Read the model definition and answer for the solid it produces. Units are mm, in the model's axes. A direction names the side the tool comes from. Give positions to 0.01 mm unless a question says otherwise; leave off trailing zeros. Write each loop counter-clockwise with the first axis right and the second up, starting at its lowest first coordinate (ties: lowest second). Pieces come first, ordered by that corner, then holes.
Solid Edge part; units mm, degrees
sketch "Sketch1" plane through (0, 0, 0) normal (0, 0, 1) x (1, 0, 0)
  circle A0 centre (0, 0) radius 41.05
  circle A1 centre (0, 0) radius 20.625
  circle A2 centre (159.79, 0) radius 23.37
  circle A3 centre (159.79, 0) radius 10
extrude "Protrusion1" add sketch "Sketch1" along normal blind 17.73
sketch "Sketch2" plane through (0, 0, 0) normal (0, 0, 1) x (1, 0, 0)
  line L0 (159.79, -23.37) -> (139.6358, 0)
  line L1 (139.6358, 0) -> (159.79, 23.37)
  line L2 (8.6959, 40.1184) -> (159.79, 23.37)
  line L3 (8.6959, 40.1184) -> (28.7283, 0)
  line L4 (28.7283, 0) -> (8.6959, -40.1184)
  line L5 (159.79, -23.37) -> (8.6959, -40.1184)
extrude "ExtrudedProtrusion_2" add sketch "Sketch2" along normal blind 12.7
sketch "Sketch3" plane through (0, 0, 0) normal (0, 0, 1) x (1, 0, 0)
  line L0 (-5.0718, -15.3845) -> (-10.7875, -12.0845)
  line L1 (-10.7875, -12.0845) -> (-13.2875, -16.4147)
  line L2 (-13.2875, -16.4147) -> (-7.5718, -19.7147)
  line L3 (-5.0718, -15.3845) -> (-7.5718, -19.7147)
  line L4 (-10.7875, 12.0845) -> (-5.0718, 15.3845)
  line L5 (-5.0718, 15.3845) -> (-7.5718, 19.7147)
  line L6 (-7.5718, 19.7147) -> (-13.2875, 16.4147)
  line L7 (-10.7875, 12.0845) -> (-13.2875, 16.4147)
  line L8 (15.8593, -3.3) -> (20.8593, -3.3)
  line L9 (20.8593, -3.3) -> (20.8593, 3.3)
  line L10 (15.8593, 3.3) -> (20.8593, 3.3)
  line L11 (15.8593, 3.3) -> (15.8593, -3.3)
extrude "Protrusion2" add sketch "Sketch3" along normal up to vertex (17.73 mm away)
Item 1: Section D-D (x = 166.5) is taken. Write down the section's boundary in (y, z), and give its area (3 significant figures).
Result set:
outline: (-22.39, 0) - (-7.41, 0) - (-7.41, 17.73) - (-22.39, 17.73) - close; (7.41, 0) - (22.39, 0) - (22.39, 17.73) - (7.41, 17.73) - close
area: 531 mm2
Item 2: Which of the six approach directions +Z, -Z, +X, -X, +Y, -Y give full straight-line access (tool end or side, diameter ignored) to faces 1 (the cylindrical face through (-41, -2, 11)), 2 (the flat face through (83.19, 31.86, 6.26)), 3 (the flat face through (-11.9, 14.01, 8.74))?
Result set:
face 1: +Z
face 2: +Z, -Z, +X, +Y
face 3: +Z, -Z
Item 3: Each of these flat-tipped pins is pushed along its axis until it touches: pin 1 Ø1.3 at (x, z) = (19, 7.5) entering from +Y; pin 2 Ø5 at (x, z) = (17.5, 6) entering from -Y; pin 3 Ø24 at (x, y) = (79.5, 12) entering from +Z. Where does it stop, or does it pass through?
Result set:
pin 1: stops at y = 39.05
pin 2: stops at y = -39.42
pin 3: stops at z = 12.7
Item 4: Find the intervals of material crossed by line 1 along X through (y, z) = (-13.5, 16.25); line 2 along X through (y, z) = (2, 4.25); line 3 along Y through (x, z) = (159.79, 10.5), in increasing order.
Result set:
line 1: x = -38.77 to -15.59, -11.6 to -8.34, 15.59 to 38.77, 140.71 to 178.87
line 2: x = -41 to -20.53, 15.86 to 149.99, 169.59 to 183.07
line 3: y = -23.37 to -10, 10 to 23.37
Item 5: Section B-B (x = 0) is taken. Write down the section's boundary in (y, z) (3 decimals), and give its area (3 significant figures).
Result set:
outline: (-41.05, 0) - (-20.625, 0) - (-20.625, 17.73) - (-41.05, 17.73) - close; (20.625, 0) - (41.05, 0) - (41.05, 17.73) - (20.625, 17.73) - close
area: 724 mm2
Item 6: Section A-A (y = 0) is taken. Write down the section's boundary in (x, z) (3 decimals).
Result set:
outline: (-41.05, 0) - (-20.625, 0) - (-20.625, 17.73) - (-41.05, 17.73) - close; (15.859, 0) - (149.79, 0) - (149.79, 17.73) - (136.42, 17.73) - (136.42, 12.7) - (41.05, 12.7) - (41.05, 17.73) - (15.859, 17.73) - close; (169.79, 0) - (183.16, 0) - (183.16, 17.73) - (169.79, 17.73) - close
Item 7: Section C-C (z = 4) is taken. Give the number of separate pieces and of enclosed holes in the cut face, and give its area (3 significant figures).
Result set:
separate pieces: 1
enclosed holes: 2
area: 12,200 mm2
Item 8: Determine the mould class of faces 4 (the flat face through (85.301, -31.627, 6.261)), 5 (the flat face through (170, 0, 17.73)), 6 (the cylindrical face through (181.38, 8.95, 10.71)) for opening direction X: pulls with the +X half, pulls with the -X half, needs draft (parallel to the pull), parting line crosses it, or undercut.
Result set:
face 4: pulls with the +X half
face 5: needs draft
face 6: undercut
